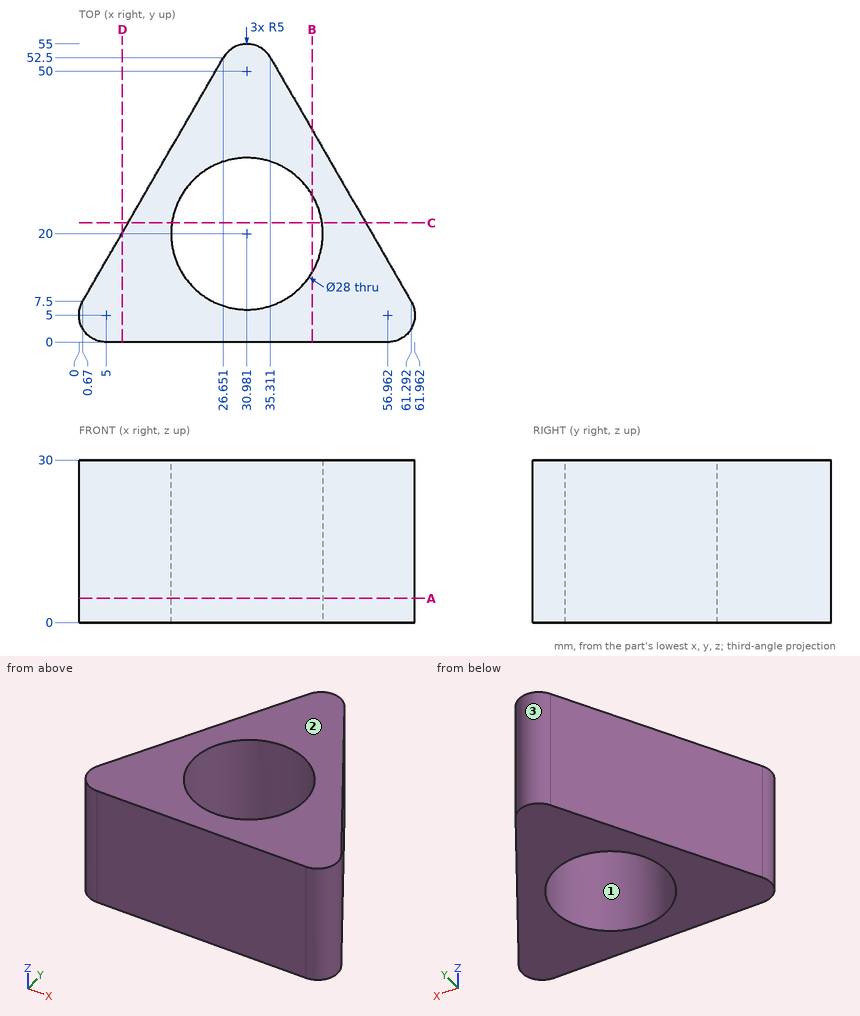
Can you work these out from the drawing? Everything is in mm from the part's minimum corner. Coordinates: 2 decimals unless noted, no trailing zeros. Loops run counter-clockwise (first coordinate to the right, second up) from the corner with the lowest first, then second, coordinate; pieces in that order, holes last. Notation, with made-up numbers: (17, 40) - (42, 40) arc R18 cw to (42, 67) - close; hole circle Ø7 at (73.25, 57.5). An arc over 180 degrees is marked (long way). Use a Markdown table: item, result.
Item 1: We'd pull the mould along X, two halves only. Please class the marked faces 1, 2 and 3: released by +X, released by -X, zero draft, split by the parting line, or undercut.
Numbers:
| item | result |
|---|---|
| face 1 | undercut |
| face 2 | zero draft |
| face 3 | split by the parting line |
Item 2: I want a section at C-C on y = 22. Please give me the cut outline in (x, z) (1 decimal), and give its area (3 significant figures).
Numbers:
| item | result |
|---|---|
| outline | (9, 0) - (17.1, 0) - (17.1, 30) - (9, 30) - close; (44.8, 0) - (52.9, 0) - (52.9, 30) - (44.8, 30) - close |
| area | 485 mm2 |
Item 3: I want a section at B-B on x = 43. Please give me the cut outline in (y, z).
Numbers:
| item | result |
|---|---|
| outline | (0, 0) - (12.82, 0) - (12.82, 30) - (0, 30) - close; (27.18, 0) - (39.18, 0) - (39.18, 30) - (27.18, 30) - close |
Item 4: Will these pins go through, and if not, where does the flat tip stop? pin 1 (3 mm diameter, centred on y = 14, z = 7, fed in from -X); pin 2 (8 mm diameter, centred on x = 20, z = 17, fed in from +Y); pin 3 (5 mm diameter, centred on y = 9.5, z = 8, fed in from -X).
Numbers:
| item | result |
|---|---|
| pin 1 | stops at x = 3.56 |
| pin 2 | stops at y = 47.91 |
| pin 3 | stops at x = 0.42 |
Item 5: I want a section at A-A on z = 4.5. Please give me the cut outline in (x, y).
Numbers:
| item | result |
|---|---|
| outline | (0.67, 7.5) arc R5 ccw to (5, 0) - (56.96, 0) arc R5 ccw to (61.29, 7.5) - (35.31, 52.5) arc R5 ccw to (26.65, 52.5) - close; hole circle Ø28 at (30.98, 20) |
Item 6: If I drill on probe 1 along Y at (x, z) = (31, 4.25); probe 2 along X at (y, z) = (8, 20.25) (1 decimal); probe 3 along Y at (x, z) = (37, 17.5) (1 decimal), over which ranges is the centre line in solid material (lowest first)? Write a range as from..to.
Numbers:
| item | result |
|---|---|
| probe 1 | y = 0..6, 34..55 |
| probe 2 | x = 1..23.8, 38.2..61 |
| probe 3 | y = 0..7.4, 32.6..49.6 |
Item 7: I want a section at D-D on x = 8. Please give me the cut outline in (y, z).
Numbers:
| item | result |
|---|---|
| outline | (0, 0) - (20.2, 0) - (20.2, 30) - (0, 30) - close |
